Part model, mm, in its own coordinate system. A direction names the side the tool comes from. Give positions to 0.01 mm unless a question says otherwise; leave off trailing zeros. Write each loop counter-clockwise with the first axis right and the second up, starting at its lowest first coordinate (ties: lowest second). Pieces come first, ordered by that corner, then holes. Notation, with made-up numbers: (19, 21.25) - (52, 21.25) arc R24 cw to (52, 46.25) - close; hole circle Ø4 at (-0.75, -9.5). An arc over 180 degrees is marked (long way). Answer in a Markdown table with one row per item. Add a question column.
1. Band-saw the part on D-D on x = 33. Write the cut outline in (y, z).
2. Band-saw the part on C-C on y = 27. Write the cut outline in (x, z).
3. Pull direction Z, two halves, no side cores. Call faces 1 (the cylindrical face through (25.645, 33.854, 2.535)), 2 (the cylindrical face through (38, 6, -2)), 3 (the flat face through (-4.75, 3, -20)), 4 (the cylindrical face through (47.44, 2.54, -12.25)): released by +Z, released by -Z, zero draft, split by the parting line, or undercut.
4. Which spindle directions (+Z, -Z, +X, -X, +Y, -Y) get a long thin tool onto all of the face, cutting with end or side? Do faces 5 (the flat face through (0, 20, 2)), 6 (the cylindrical face through (12.157, 5.798, -1.377)), 7 (the flat face through (40, 20, 2)). Say none if no direction does.
5. Band-saw the part on B-B on z = -19. Write the cut outline in (x, y), plus the area to 3 significant figures.
6. Drop flat-ended pins along their axis: pin 1 Ø19 at (x, y) = (20, 25) entering from -Z; pin 2 Ø5.5 at (y, z) = (20, 3) entering from -X; pin 3 Ø4 at (y, z) = (22, 2) entering from +X; pin 4 Ø10 at (x, y) = (-1.5, 24) entering from -Z. Give the stop position or say it passes through.
7. Probe line 1 along Y through (x, z) = (20, 2.1); line 2 along X through (y, z) = (3, -20.5); line 3 along Z through (x, y) = (4, 34.5). List the from-to ranges inside material, lowest first.
8. Band-saw the part on A-A on x = 20. Write the cut outline in (y, z), plus the area to 3 significant figures.
```python
from build123d import *

# Parameters (mm, degrees)
SKETCH1_W           = 40
SKETCH1_H           = 30
BOSS_EXTRUDE1_DEPTH = 5
BOSS_EXTRUDE2_DEPTH = 5
SKETCH4_R           = 10.5
SKETCH4_R_2         = 1.6
CUT_EXTRUDE2_DEPTH  = 5
SKETCH5_W           = 15
SKETCH5_H           = 30
BOSS_EXTRUDE3_DEPTH = 5
CHAMFER1_SIZE       = 5
CHAMFER1_SIZE_2     = 28.356409098
CHAMFER2_SIZE       = 5
CHAMFER2_SIZE_2     = 28.356409098
FILLET1_R           = 10
FILLET2_R           = 5
FILLET4_R           = 5
CUT_EXTRUDE3_DEPTH  = 78.136243103


with BuildPart() as part:
    # Sketch1 → Boss-Extrude1 (new body)
    with BuildSketch(Plane(origin=(0, 0, 0), x_dir=(1, 0, 0), z_dir=(0, 1, 0))):
        with Locations((20, 15)):
            Rectangle(SKETCH1_W, SKETCH1_H)
    extrude(amount=BOSS_EXTRUDE1_DEPTH)

    # Sketch2 → Boss-Extrude2 (add)
    with BuildSketch(Plane.XY):
        with BuildLine():
            Line((0, 5), (0, 25))
            ThreePointArc((0, 25), (20, 45), (40, 25))
            Line((40, 25), (40, 5))
            Line((40, 5), (40, 0))
            Line((40, 0), (0, 0))
            Line((0, 0), (0, 5))
        make_face()
    extrude(amount=BOSS_EXTRUDE2_DEPTH)

    # Sketch4 → Cut-Extrude2 (cut)
    with BuildSketch(Plane.XY.offset(5)):
        with Locations((20, 25)):
            Circle(SKETCH4_R)
        with Locations((20, 40.011106999)):
            Circle(SKETCH4_R_2)
        with Locations((7, 17.494446501)):
            Circle(SKETCH4_R_2)
        with Locations((33, 17.494446501)):
            Circle(SKETCH4_R_2)
    extrude(amount=-CUT_EXTRUDE2_DEPTH, mode=Mode.SUBTRACT)

    # Sketch5 → Boss-Extrude3 (add)
    # profile 1 of 2: a face of its own
    with BuildSketch(Plane(origin=(0, 5, 0), x_dir=(1, 0, 0), z_dir=(0, 1, 0))):
        with Locations((-7.5, 15)):
            Rectangle(SKETCH5_W, SKETCH5_H)
        with BuildLine():
            Line((-10.25, 15), (-10.25, 25))
            ThreePointArc((-10.25, 25), (-7.5, 27.75), (-4.75, 25))
            Line((-4.75, 25), (-4.75, 15))
            ThreePointArc((-4.75, 15), (-7.5, 12.25), (-10.25, 15))
        make_face(mode=Mode.SUBTRACT)
    # profile 2 of 2: a face of its own
    with BuildSketch(Plane(origin=(0, 5, 0), x_dir=(1, 0, 0), z_dir=(0, 1, 0))):
        with Locations((47.5, 15)):
            Rectangle(SKETCH5_W, SKETCH5_H)
        with BuildLine():
            Line((50.25, 15), (50.25, 25))
            ThreePointArc((50.25, 25), (47.5, 27.75), (44.75, 25))
            Line((44.75, 25), (44.75, 15))
            ThreePointArc((44.75, 15), (47.5, 12.25), (50.25, 15))
        make_face(mode=Mode.SUBTRACT)
    extrude(amount=-BOSS_EXTRUDE3_DEPTH)

    # Chamfer1
    # the kernel refuses this chamfer: 28.356409098, 5 mm, written as the material it adds along each edge
    with BuildSketch(Plane(origin=(0, 5, 0), x_dir=(0.21013876076743523, 0, 0.9776715712462578), z_dir=(0, -1, 0))) as chamfer1_piece_1_section:
        Polygon((CHAMFER1_SIZE * 0.977671571246, CHAMFER1_SIZE * 0.210138760767), (-CHAMFER1_SIZE_2 * 0.210138760768, CHAMFER1_SIZE_2 * 0.977671571249), (0, 0), align=None)
    chamfer1_piece_1 = extrude(amount=5, mode=Mode.PRIVATE)
    chamfer1_piece_1 = split(chamfer1_piece_1, bisect_by=Plane(origin=(-6.173112567, 2.5, 5), z_dir=(0, 0, -1)), keep=Keep.TOP, mode=Mode.PRIVATE)
    chamfer1_piece_1 = split(chamfer1_piece_1, bisect_by=Plane(origin=(-15, 2.5, 1.987176297), z_dir=(1, 0, 0)), keep=Keep.TOP, mode=Mode.PRIVATE)
    add(chamfer1_piece_1)

    # Chamfer2
    # the kernel refuses this chamfer: 28.356409098, 5 mm, written as the material it adds along each edge
    with BuildSketch(Plane(origin=(40, 5, 0), x_dir=(-0.2101387607674354, 0, 0.9776715712462578), z_dir=(0, -1, 0))) as chamfer2_piece_1_section:
        Polygon((CHAMFER2_SIZE * 0.977671571246, -CHAMFER2_SIZE * 0.210138760767), (-CHAMFER2_SIZE_2 * 0.210138760768, -CHAMFER2_SIZE_2 * 0.977671571249), (0, 0), align=None)
    chamfer2_piece_1 = extrude(amount=5, mode=Mode.PRIVATE)
    chamfer2_piece_1 = split(chamfer2_piece_1, bisect_by=Plane(origin=(46.173112567, 2.5, 5), z_dir=(0, 0, -1)), keep=Keep.TOP, mode=Mode.PRIVATE)
    chamfer2_piece_1 = split(chamfer2_piece_1, bisect_by=Plane(origin=(55, 2.5, 1.987176297), z_dir=(-1, 0, 0)), keep=Keep.TOP, mode=Mode.PRIVATE)
    add(chamfer2_piece_1)

    # Fillet1
    fillet1_edges = [part.edges().sort_by_distance(p)[0] for p in [
        (40, 5, 2.5),
        (0, 5, 2.5),
    ]]
    fillet(fillet1_edges, radius=FILLET1_R)

    # Fillet2
    fillet2_edges = [part.edges().sort_by_distance(p)[0] for p in [
        (55, 2.5, 2.355095289),
        (-15, 2.5, -30),
        (55, 2.5, -30),
        (-15, 2.5, 2.355095289),
    ]]
    fillet(fillet2_edges, radius=FILLET2_R)

    # Fillet4
    fillet4_edges = [part.edges().sort_by_distance(p)[0] for p in [
        (20, 5, 0),
    ]]
    fillet(fillet4_edges, radius=FILLET4_R)

    # Sketch6 → Cut-Extrude3 (cut, through all)
    with BuildSketch(Plane(origin=(0, 0, 0), x_dir=(-1, 0, 0), z_dir=(0, 0, -1))):
        with BuildLine():
            Line((-25.611038109, 5), (-14.388961891, 5))
            ThreePointArc((-14.388961891, 5), (-3.752498092, 12.523671995), (0, 25))
            ThreePointArc((0, 25), (-20, 45), (-40, 25))
            ThreePointArc((-40, 25), (-36.247501908, 12.523671995), (-25.611038109, 5))
        make_face()
    extrude(amount=CUT_EXTRUDE3_DEPTH, mode=Mode.SUBTRACT)


solid = part.part
```
Values:
| question | item | result |
|---|---|---|
| 1 | outline | (0, -30) - (5, -30) - (5, -5) arc R5 cw to (8.99, -0.1) - (8.99, 0) - (15.89, 0) - (15.89, 5) - (0, 5) - close; (19.09, 0) - (40.2, 0) - (40.2, 5) - (19.09, 5) - close |
| 2 | outline | (0.1, 0) - (9.69, 0) - (9.69, 5) - (0.1, 5) - close; (30.31, 0) - (39.9, 0) - (39.9, 5) - (30.31, 5) - close |
| 3 | face 1 | zero draft |
| 3 | face 2 | released by -Z |
| 3 | face 3 | undercut |
| 3 | face 4 | undercut |
| 4 | face 5 | +Z, -Z, -X, +Y |
| 4 | face 6 | -Z, +Y |
| 4 | face 7 | +Z, -Z, +X, +Y |
| 5 | outline | (-15, 0) - (-10.25, 0) - (-10.25, 5) - (-15, 5) - close; (-4.75, 0) - (44.75, 0) - (44.75, 5) - (-4.75, 5) - close; (50.25, 0) - (55, 0) - (55, 5) - (50.25, 5) - close |
| 5 | area | 295 mm² |
| 6 | pin 1 | passes through |
| 6 | pin 2 | stops at x = 0 |
| 6 | pin 3 | stops at x = 40 |
| 6 | pin 4 | stops at z = 0 |
| 7 | line 1 | y = 0 to 14.5, 35.5 to 38.41, 41.61 to 45 |
| 7 | line 2 | x = -15 to -10.25, -4.75 to 44.75, 50.25 to 55 |
| 7 | line 3 | z = 0 to 5 |
| 8 | outline | (0, -30) - (5, -30) - (5, 0) - (14.5, 0) - (14.5, 5) - (0, 5) - close; (35.5, 0) - (38.41, 0) - (38.41, 5) - (35.5, 5) - close; (41.61, 0) - (45, 0) - (45, 5) - (41.61, 5) - close |
| 8 | area | 254 mm² |
